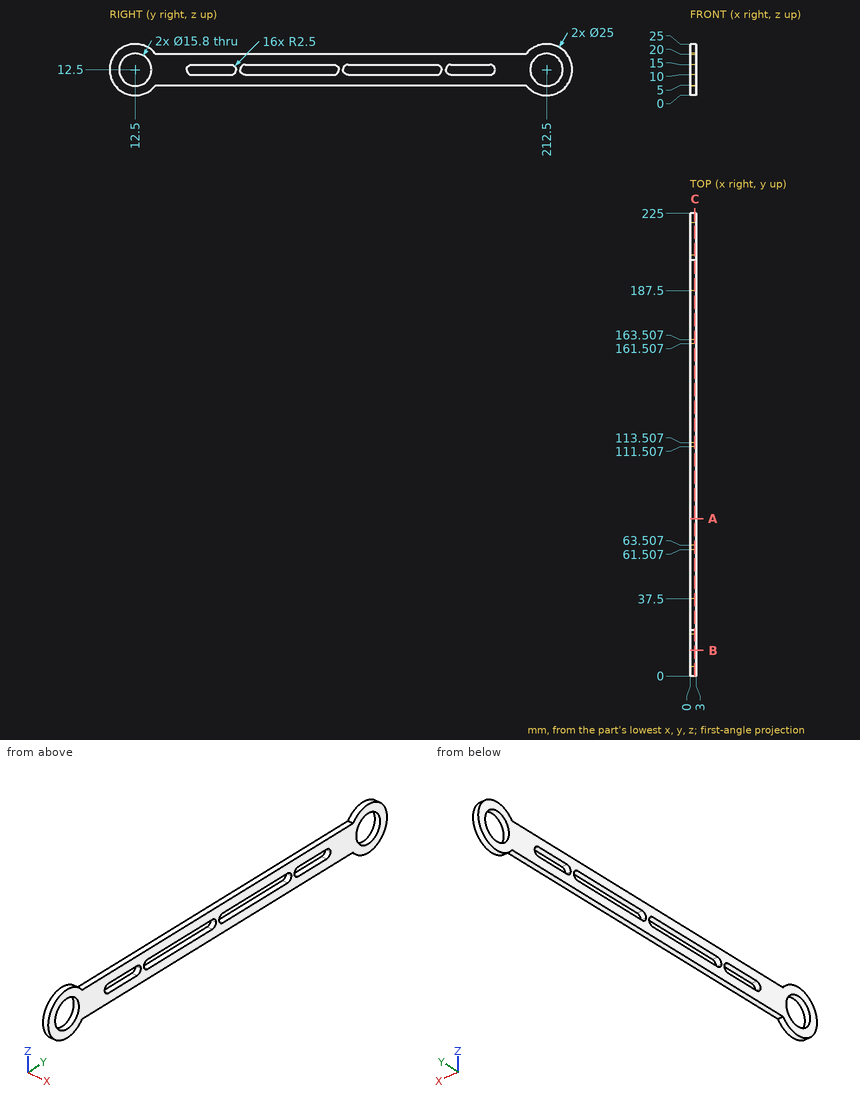
The figure shows three views and two pictorial views of one solid part (mm, origin at its lowest corner). Answer the questions. Coordinates: 2 decimals unless noted, no trailing zeros. Loops run counter-clockwise (first coordinate to the right, second up) from the corner with the lowest first, then second, coordinate; pieces in that order, holes last. Notation, with made-up numbers: (16.25, 35.25) - (35.25, 35.25) arc R20 ccw to (35.25, 62.25) - close; hole circle Ø2 at (0, 60). An arc over 180 degrees is marked (long way). Use a Markdown table: item, result. Add a question column.
1) Given pin 1 (1 mm diameter, centred on x = 2.5, y = 47.5, fed in from +Z); pin 2 (0.9 mm diameter, centred on x = 1.5, y = 124, fed in from -Z); pin 3 (1 mm diameter, centred on x = 1.5, z = 6, fed in from -Y), each flat-ended and moving along its own axis, determine where each tip first touches the part or whether it passes through.
2) Find the intervals of material crossed by line 1 (Z direction, x = 1.8, y = 85); line 2 (Y direction, x = 2.95, z = 19.75); line 3 (Y direction, x = 2.4, z = 18.25), in increasing order.
3) The part is cut by section A-A, the plane y = 76.5. Give the vertices of the cut face in (x, z), and give its area (3 significant figures).
4) The part is cut by section B-B, the plane y = 12.5. Give the vertices of the cut face in (x, z).
5) The part is cut by section C-C, the plane x = 2.25. State how many separate pieces and enclosed holes the cut face has, and give its area (3 significant figures).
Here are the results:
| question | item | result |
|---|---|---|
| 1 | pin 1 | stops at z = 20 |
| 1 | pin 2 | stops at z = 5 |
| 1 | pin 3 | stops at y = 1.53 |
| 2 | line 1 | z = 5 to 10, 15 to 20 |
| 2 | line 2 | y = 2.32 to 9.36, 15.64 to 209.36, 215.64 to 222.68 |
| 2 | line 3 | y = 1.4 to 7.08, 17.92 to 207.08, 217.92 to 223.6 |
| 3 | outline | (0, 5) - (3, 5) - (3, 10) - (0, 10) - close; (0, 15) - (3, 15) - (3, 20) - (0, 20) - close |
| 3 | area | 30.0 mm^2 |
| 4 | outline | (0, 0) - (3, 0) - (3, 4.6) - (0, 4.6) - close; (0, 20.4) - (3, 20.4) - (3, 25) - (0, 25) - close |
| 5 | separate pieces | 1 |
| 5 | enclosed holes | 6 |
| 5 | area | 2,540 mm^2 |
